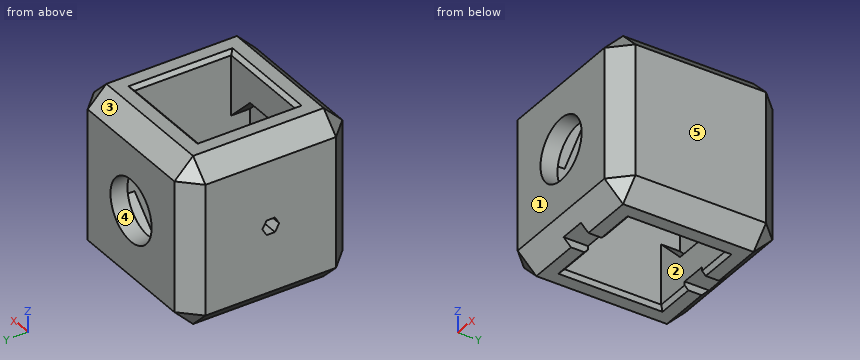
from build123d import *

# Parameters (mm, degrees)
F0_W      = 45
F0_H      = 45
F0_W_2    = 25.9
F0_H_2    = 25.9
F1_DEPTH  = 45
F2_R      = 8.3
F3_DEPTH  = 45.001
F5_DEPTH  = 5
F7_DEPTH  = 5
F9_SIZE   = 5
F10_DEPTH = 9.55
F11_SIZE  = 1
F12_W     = 7
F12_H     = 60
F13_DEPTH = 2


# Not quite as in the source:
# - a feature names something its author has since deleted; it is built from what else it names


with BuildPart() as f1:
    # F0 (on Top) → F1 (new body)
    with BuildSketch(Plane.XY):
        Rectangle(F0_W, F0_H)
        Rectangle(F0_W_2, F0_H_2, mode=Mode.SUBTRACT)
    extrude(amount=F1_DEPTH)

    # F2 (on face) → F3 (cut, through all)
    with BuildSketch(Plane.XZ.offset(22.5)):
        with Locations((0, 22.5)):
            Circle(F2_R)
    extrude(amount=-F3_DEPTH, mode=Mode.SUBTRACT)

    # F4 (on face) → F5 (cut)
    with BuildSketch(Plane.XZ.offset(-12.95)):
        Polygon((12.95, 17.1359343673), (12.95, 27.8640656327), (5.3640656327, 35.45), (-5.3640656327, 35.45), (-12.95, 27.8640656327), (-12.95, 17.1359343673), (-5.3640656327, 9.55), (5.3640656327, 9.55), align=None)
    extrude(amount=-F5_DEPTH, mode=Mode.SUBTRACT)

    # F6 (on face) → F7 (cut)
    with BuildSketch(Plane(origin=(0, -12.95, 0), x_dir=(-1, 0, 0), z_dir=(0, 1, 0))):
        Polygon((12.95, 17.1359343673), (12.95, 27.8640656327), (5.3640656327, 35.45), (-5.3640656327, 35.45), (-12.95, 27.8640656327), (-12.95, 17.1359343673), (-5.3640656327, 9.55), (5.3640656327, 9.55), align=None)
    extrude(amount=-F7_DEPTH, mode=Mode.SUBTRACT)

    # F9
    f9_edges = [f1.edges().sort_by_distance(p)[0] for p in [
        (22.5, -22.5, 22.5),
        (22.5, 22.5, 22.5),
        (22.5, 0, 0),
        (22.5, 0, 45),
        (-22.5, 22.5, 22.5),
        (-22.5, -22.5, 22.5),
        (-22.5, 0, 0),
        (-22.5, 0, 45),
        (0, -22.5, 0),
        (0, -22.5, 45),
        (0, 22.5, 45),
        (0, 22.5, 0),
    ]]
    chamfer(f9_edges, length=F9_SIZE)

    # F8 (on face) → F10 (cut, through all)
    with BuildSketch(Plane(origin=(-22.5, 0, 0), x_dir=(0, -1, 0), z_dir=(-1, 0, 0))):
        Polygon((1.1258330249, 20.55), (2.2516660498, 22.5), (1.1258330249, 24.45), (-1.1258330249, 24.45), (-2.2516660498, 22.5), (-1.1258330249, 20.55), align=None)
    extrude(amount=-F10_DEPTH, mode=Mode.SUBTRACT)

    # F11
    f11_edges = [f1.edges().sort_by_distance(p)[0] for p in [
        (12.95, 0, 45),
        (0, -12.95, 45),
        (-12.95, 0, 45),
        (0, 12.95, 45),
        (-12.95, 0, 0),
        (0, 12.95, 0),
        (12.95, 0, 0),
        (0, -12.95, 0),
    ]]
    chamfer(f11_edges, length=F11_SIZE)

    # F12 (on face) → F13 (cut)
    with BuildSketch(Plane(origin=(0, 0, 0), x_dir=(1, 0, 0), z_dir=(0, 0, -1))):
        Rectangle(F12_W, F12_H)
    extrude(amount=-F13_DEPTH, mode=Mode.SUBTRACT)


solid = f1.part
Read the model definition and answer for the solid it produces. Units are mm, in the model's axes. Face numbers are marked on the shaded views. A direction names the side the tool comes from. Round coordinates to 2 decimals unless told otherwise and drop trailing zeros. Loops run counter-clockwise (first coordinate to the right, second up) from the corner with the lowest first, then second, coordinate; pieces in that order, holes last.
Q1. Which of the six approach directions +Z, -Z, +X, -X, +Y, -Y give full straight-line access (tool end or side, diameter ignored) to the marked faces 1 and 2?
Q2. Section C-C on z = 8 is taken. Write down the section's boundary in (x, y).
Q3. Consider probe 1 along X at (y, z) = (-12.5, 8). Determine where the line is inside the solid, lowest interval first.
Q4. Section A-A on y = -11 is taken. Write down the section's boundary in (x, z).
Q5. Section B-B on x = 0 is taken. Give the number of separate pieces and of enclosed holes in the cut face, and give its area (3 significant figures).
Q6. Section D-D on x = 16.5 is taken. Write down the section's boundary in (y, z).
Q7. Each of these flat-tipped pins is pushed along its axis until it touches: pin 1 (5.5 mm diameter, centred on x = -2, y = -15.5, fed in from -Z); pin 2 (0.7 mm diameter, centred on x = -20, y = -0.5, fed in from +Z); pin 3 (1.5 mm diameter, centred on x = 2.5, y = 15, fed in from -Z); pin 4 (0.6 mm diameter, centred on y = -16.5, z = 1, fed in from +X). Where does it stop, or does it pass through?
Q8. Determine the mould class of the marked faces 3, 4 and 5 for opening direction X: released by +X, released by -X, zero draft, split by the parting line, or undercut.
Output:
1. face 1: +Z, -Z, +X, -X, -Y
1. face 2: +Z, -Z
2. outline: (-22.5, -17.5) - (-17.5, -22.5) - (17.5, -22.5) - (22.5, -17.5) - (22.5, 17.5) - (17.5, 22.5) - (-17.5, 22.5) - (-22.5, 17.5) - close; hole (-12.95, -12.95) - (12.95, -12.95) - (12.95, 12.95) - (-12.95, 12.95) - close
3. probe 1: x = -22.5 to -12.95, 12.95 to 22.5
4. outline: (-22.5, 5) - (-17.5, 0) - (-13.95, 0) - (-12.95, 1) - (-12.95, 44) - (-13.95, 45) - (-17.5, 45) - (-22.5, 40) - close; (12.95, 1) - (13.95, 0) - (17.5, 0) - (22.5, 5) - (22.5, 40) - (17.5, 45) - (13.95, 45) - (12.95, 44) - close
5. separate pieces: 4
5. enclosed holes: 0
5. area: 376 mm2
6. outline: (-22.5, 5) - (-17.5, 0) - (17.5, 0) - (22.5, 5) - (22.5, 40) - (17.5, 45) - (-17.5, 45) - (-22.5, 40) - close
7. pin 1: stops at z = 0
7. pin 2: stops at z = 42.85
7. pin 3: stops at z = 2
7. pin 4: stops at x = 18.8
8. face 3: zero draft
8. face 4: undercut
8. face 5: released by +X
